Design review of the part built by this model. Coordinates are the model's own, in mm. A direction names the side the tool comes from. Give positions to 0.01 mm unless a question says otherwise; leave off trailing zeros. Write each loop counter-clockwise with the first axis right and the second up, starting at its lowest first coordinate (ties: lowest second). Pieces come first, ordered by that corner, then holes. Notation, with made-up numbers: M -6,-36 L 53,-36 A24 ccw 53,-19 Z; hole C 81,-40 d6. An arc over 180 degrees is marked long. One line per item, written item: value. Start each with the question number.
```python
from build123d import *

# Parameters (mm, degrees)
EXTRUDE1_DEPTH = 3.5


with BuildPart() as part:
    # Sketch1 → Revolve1 (revolve)
    with BuildSketch(Plane.XY, mode=Mode.PRIVATE) as revolve1_sk:
        Polygon((-201.999999982, -47.5), (201.999999982, -47.5), (401.999999982, -46.75), (402.999999982, -45.742471769), (402.999999982, -16.5), (406.999999982, -16.5), (407.999999982, -15.5), (407.999999982, -12.5), (432.999999982, -12.5), (433.999999982, -11.5), (433.999999982, -10), (502.999999982, -10), (503.999999982, -9), (503.999999982, 0), (-425.999999982, 0), (-425.999999982, -11.5), (-424.999999982, -12.5), (-407.999999982, -12.5), (-407.999999982, -15.5), (-406.999999982, -16.5), (-402.999999982, -16.5), (-402.999999982, -45.75), (-401.999999982, -46.75), align=None)
    revolve(revolve1_sk.sketch.rotate(Axis((-425.999999982, 0, 0), (1, 0, 0)), 270), axis=Axis((-425.999999982, 0, 0), (1, 0, 0)))  # turned: the seam where the file's is

    # Sketch2 → Extrude1 (cut)
    with BuildSketch(Plane(origin=(468.499999982, 0, -10), x_dir=(0, -1, 0), z_dir=(0, 0, -1))):
        with BuildLine():
            Line((-3, 16.5), (-3, -27.5))
            ThreePointArc((-3, -27.5), (0, -30.5), (3, -27.5))
            Line((3, -27.5), (3, 16.5))
            ThreePointArc((3, 16.5), (0, 19.5), (-3, 16.5))
        make_face()
    extrude(amount=-EXTRUDE1_DEPTH, mode=Mode.SUBTRACT)


solid = part.part
```
Q1. Take a section at A-A, the plane x = 123.5. Give the boundary of the cut face in (y, z), then the cut area to 3 significant figures.
Q2. Wall thickness on line 1 (X direction, y = -7, z = 41.5); line 2 (Y direction, x = -70, z = 2); line 3 (X direction, y = -27, z = 37): over which ranges is each line inside the solid? List them lowest first. Write a range as from..to.
Q3. For P1, Ø4, axis at x = 264, y = 31.5, coming from the -Z side; P2, Ø5, axis at x = 246.5, z = 26.5, coming from the -Y side; P3, Ø1.5, axis at x = 476.5, z = -8, coming from the +Y side, all flat-tipped, find the tip position at first contact; note any pin that passes through.
Q4. Take a section at B-B, the plane x = 220. Give the boundary of the cut face in (y, z) (1 decimal), then the cut area to 3 significant figures.
Q5. Machinability: for faces 1 (the face through (-403, -1, -20)), 2 (the face through (504, 0, 0)), 3 (the face through (303.4, 46, -10.21)), which of the approach directions +Z, -Z, +X, -X, +Y, -Y give a long, thin tool a straight path to every point of the face, cutting with its end or side? Answer none if there is none.
Results list:
1. outline: C 0,0 d95
1. area: 7,090 mm^2
2. line 1: x = -403..403
2. line 2: y = -47.46..47.46
2. line 3: x = -402.95..402.94
3. P1: stops at z = -36.93
3. P2: stops at y = -40.8
3. P3: stops at y = 6.89
4. outline: C 0,0 d94.9
4. area: 7,070 mm^2
5. face 1: -X
5. face 2: +Z, -Z, +X, +Y, -Y
5. face 3: +X
